The listing builds one solid part. Answer for the finished solid, in the listing's coordinates (mm). A direction names the side the tool comes from. Give positions to 0.01 mm unless a question says otherwise; leave off trailing zeros. Write each loop counter-clockwise with the first axis right and the second up, starting at its lowest first coordinate (ties: lowest second). Pieces come first, ordered by that corner, then holes. Notation, with made-up numbers: (-30, -29.5) - (11, -29.5) arc R26 cw to (11, 2.5) - close; hole circle Ø6 at (1, 54). An arc over 180 degrees is marked (long way). One line per item, written item: value. Start each with the question number.
from build123d import *

# Parameters (mm, degrees)
SKETCH1_W                       = 104.5
SKETCH1_H                       = 59.5
BOSS_EXTRUDE1_DEPTH             = 10
BOSS_EXTRUDE2_REACH             = 62.952
BOSS_EXTRUDE2_DIRECTION_2_REACH = 62.952
SKETCH4_W                       = 20
SKETCH4_H                       = 8.6
SKETCH4_H_2                     = 8.7
CUT_EXTRUDE1_DEPTH              = 66.116242213
M4_CLEARANCE_HOLE1_D            = 4.8
BOSS_EXTRUDE3_REACH             = 71.571
BOSS_EXTRUDE3_DIRECTION_2_DEPTH = 120


with BuildPart() as part:
    # Sketch1 → Boss-Extrude1 (new body)
    with BuildSketch(Plane(origin=(0, 0, 0), x_dir=(1, 0, 0), z_dir=(0, 1, 0))):
        Rectangle(SKETCH1_W, SKETCH1_H)
    extrude(amount=BOSS_EXTRUDE1_DEPTH)

    # Boss-Extrude2: up to this face of the body (flat: up to its plane)
    boss_extrude2_end = Plane(part.part.faces().sort_by_distance((0, 5, 29.75))[0])
    # Sketch3 → Boss-Extrude2 (add, up to the picked face)
    with BuildSketch(Plane.XY, mode=Mode.PRIVATE) as boss_extrude2_sk1:
        with BuildLine():
            Line((52.25, 10), (52.25, 25))
            ThreePointArc((52.25, 25), (42.25, 35), (32.25, 25))
            Line((32.25, 25), (32.25, 10))
            Line((32.25, 10), (52.25, 10))
        make_face()
    boss_extrude2_tool1 = split(extrude(boss_extrude2_sk1.sketch, amount=BOSS_EXTRUDE2_REACH, mode=Mode.PRIVATE), bisect_by=boss_extrude2_end, keep=Keep.BOTH, mode=Mode.PRIVATE)
    add(boss_extrude2_tool1.solids().sort_by(Axis((42.25, 21.535979, 0), (0, 0, 1)))[0])

    # Boss-Extrude2 direction 2: up to this face of the body (flat: up to its plane)
    boss_extrude2_direction_2_end = Plane(part.part.faces().sort_by_distance((0, 5, -29.75))[0])
    # Sketch3 → Boss-Extrude2 direction 2 (add, up to the picked face)
    with BuildSketch(Plane.XY, mode=Mode.PRIVATE) as boss_extrude2_direction_2_sk1:
        with BuildLine():
            Line((52.25, 10), (52.25, 25))
            ThreePointArc((52.25, 25), (42.25, 35), (32.25, 25))
            Line((32.25, 25), (32.25, 10))
            Line((32.25, 10), (52.25, 10))
        make_face()
    boss_extrude2_direction_2_tool1 = split(extrude(boss_extrude2_direction_2_sk1.sketch, amount=-BOSS_EXTRUDE2_DIRECTION_2_REACH, mode=Mode.PRIVATE), bisect_by=boss_extrude2_direction_2_end, keep=Keep.BOTH, mode=Mode.PRIVATE)
    add(boss_extrude2_direction_2_tool1.solids().sort_by(Axis((42.25, 21.535979, 0), (0, 0, -1)))[0])

    # Sketch4 → Cut-Extrude1 (cut, through all)
    with BuildSketch(Plane(origin=(0, 10, 0), x_dir=(1, 0, 0), z_dir=(0, 1, 0))):
        with Locations((42.25, 25.45)):
            Rectangle(SKETCH4_W, SKETCH4_H)
        with Locations((42.25, 8.5)):
            Rectangle(SKETCH4_W, SKETCH4_H_2)
        with Locations((42.25, -8.5)):
            Rectangle(SKETCH4_W, SKETCH4_H_2)
        with Locations((42.25, -25.45)):
            Rectangle(SKETCH4_W, SKETCH4_H)
    extrude(amount=CUT_EXTRUDE1_DEPTH, mode=Mode.SUBTRACT)

    # M4 Clearance Hole1 (through all)
    with Locations(Plane.XY.offset(29.75)):
        with Locations((42.25, 25)):
            Hole(M4_CLEARANCE_HOLE1_D / 2)

    # Boss-Extrude3: up to this face of the body (flat: up to its plane)
    boss_extrude3_end = Plane(part.part.faces().sort_by_distance((52.25, 9.820598864, 0))[0])
    # Sketch8 → Boss-Extrude3 (add, up to the picked face)
    with BuildSketch(Plane(origin=(0, 0, 0), x_dir=(0, 0, -1), z_dir=(1, 0, 0)), mode=Mode.PRIVATE) as boss_extrude3_sk1:
        Polygon((-7, 0), (-7, -8), (-13, -14), (-13, -16), (13, -16), (13, -14), (7, -8), (7, 0), align=None)
    boss_extrude3_tool1 = split(extrude(boss_extrude3_sk1.sketch, amount=BOSS_EXTRUDE3_REACH, mode=Mode.PRIVATE), bisect_by=boss_extrude3_end, keep=Keep.BOTH, mode=Mode.PRIVATE)
    add(boss_extrude3_tool1.solids().sort_by(Axis((0, -9.098592, 0), (1, 0, 0)))[0])

    # Sketch8 → Boss-Extrude3 direction 2 (add)
    with BuildSketch(Plane(origin=(0, 0, 0), x_dir=(0, 0, -1), z_dir=(1, 0, 0))):
        Polygon((-7, 0), (-7, -8), (-13, -14), (-13, -16), (13, -16), (13, -14), (7, -8), (7, 0), align=None)
    extrude(amount=-BOSS_EXTRUDE3_DIRECTION_2_DEPTH)


solid = part.part
Item 1: Find section C-C on x = -103. Determine the outline of the cut face in (y, z), plus the area to 3 significant figures.
Item 2: Find section B-B on y = 15.5. Determine the outline of the cut face in (x, z), plus the area to 3 significant figures.
Item 3: Each of these flat-tipped pins is pushed along its axis until it touches: pin 1 Ø22 at (x, y) = (44.5, 18.5) entering from -Z; pin 2 Ø2.5 at (y, z) = (20, -1.5) entering from -X; pin 3 Ø8 at (x, z) = (9, 18.5) entering from -Y; pin 4 Ø1 at (x, y) = (-13.5, -15) entering from -Z. Where does it stop, or does it pass through?
Item 4: Find section A-A on z = 15. Determine the outline of the cut face in (x, y).
Item 5: For faces 4 (the flat face through (-1, 0, 18)), 5 (the flat face through (42, 22, -21.15)), 6 (the flat face through (42, 22, 21.15)), 7 (the flat face through (32.25, 18, 0)), 8 (the flat face through (42, 22, 12.85)), determine the directions among +Z, -Z, +X, -X, +Y, -Y from which every point of the face is accessible in a straight line to the end or side of a thin tool.
Item 6: Find section D-D on x = 42.25. Give the number of separate pieces and of enclosed holes in the cut face, plus the area to 3 significant figures.
Item 7: Straight lines are drawn through the part: line 1 along Y through (x, z) = (42.25, 0.25); line 2 along Y through (x, z) = (42, -18); line 3 along Z through (x, y) = (39.5, -2). For each, find the intervals that lie inside material, in ascending order.
Item 8: The mould has two halves that part along X. Classify faces 1 (the cylindrical face through (42.77, 22.657, 16.942)), 2 (the flat face through (-120, -10, 0)), 3 (the flat face through (-1, 0, -19)): +X half, -X half, draft (parallel to the pull), parting line (faces both ways), or undercut.
Values:
1. outline: (-16, -13) - (-14, -13) - (-8, -7) - (0, -7) - (0, 7) - (-8, 7) - (-14, 13) - (-16, 13) - close
1. area: 284 mm^2
2. outline: (32.25, -21.15) - (52.25, -21.15) - (52.25, -12.85) - (32.25, -12.85) - close; (32.25, -4.15) - (52.25, -4.15) - (52.25, 4.15) - (32.25, 4.15) - close; (32.25, 12.85) - (52.25, 12.85) - (52.25, 21.15) - (32.25, 21.15) - close
2. area: 498 mm^2
3. pin 1: z = -29.75
3. pin 2: x = 32.25
3. pin 3: y = 0
3. pin 4: z = -13
4. outline: (-52.25, 0) - (52.25, 0) - (52.25, 25) arc R10 ccw to (32.25, 25) - (32.25, 10) - (-52.25, 10) - close; hole circle Ø4.8 at (42.25, 25)
5. face 4: +Z, +X, -X
5. face 5: -Z, +X, -X, +Y
5. face 6: +Z, +X, -X, +Y
5. face 7: +Z, -Z, -X, +Y
5. face 8: +X, -X, +Y
6. separate pieces: 4
6. enclosed holes: 0
6. area: 1,380 mm^2
7. line 1: -16 to 22.6, 27.4 to 35
7. line 2: 0 to 22.61, 27.39 to 35
7. line 3: -7 to 7
8. face 1: undercut
8. face 2: -X half
8. face 3: draft
